Build history of the part. All positions in model axes, mm. Face numbers are marked on the shaded views. A direction names the side the tool comes from. Round coordinates to 2 decimals unless told otherwise and drop trailing zeros. Write each loop counter-clockwise with the first axis right and the second up, starting at its lowest first coordinate (ties: lowest second). Pieces come first, ordered by that corner, then holes. Notation, with made-up numbers: (86.5, 2.25) -> (138.5, 2.25) arc R24 ccw to (138.5, 15.25) -> close; hole circle Ø11 at (40.25, -15.75). An arc over 180 degrees is marked (long way). Return JSON: item names as keys, results as strings.
from build123d import *

# Parameters (mm, degrees)
BOSS_EXTRUDE1_DEPTH = 2.9591
SWEEP1_PROFILE_R    = 2.9591
SWEEP2_PROFILE_R    = 2.9591


with BuildPart() as part:
    # Sketch1 → Boss-Extrude1 (new, symmetric)
    with BuildSketch(Plane(origin=(0, 0, 0), x_dir=(1, 0, 0), z_dir=(0, 1, 0))):
        Polygon((7.97759508, 13.8176), (-7.97759508, 13.8176), (-15.955190159, 0), (-7.97759508, -13.8176), (7.97759508, -13.8176), (15.955190159, 0), align=None)
        Polygon((8.62284174, 0), (4.31142087, 7.4676), (-4.31142087, 7.4676), (-8.62284174, 0), (-4.31142087, -7.4676), (4.31142087, -7.4676), align=None, mode=Mode.SUBTRACT)
    extrude(amount=BOSS_EXTRUDE1_DEPTH, both=True)

    # Sweep1: sweep along a path in Sketch6
    with BuildLine(Plane(origin=(0, 0, 0), x_dir=(1, 0, 0), z_dir=(0, 1, 0))) as sweep1_path:
        Line((0, -13.8176), (0, -49.8856))
    # Sweep1 profile (on start of the path) → Sweep1 (sweep)
    with BuildSketch(Plane.XY.offset(13.8176)):
        Circle(SWEEP1_PROFILE_R)
    sweep(path=sweep1_path.line)

    # Sweep2: sweep along a path in Sketch6<4>
    with BuildLine(Plane(origin=(0, 0, 0), x_dir=(1, 0, 0), z_dir=(0, 1, 0))) as sweep2_path:
        Line((25.4, -49.8856), (-25.4, -49.8856))
    # Sweep2 profile (on start of the path) → Sweep2 (sweep)
    with BuildSketch(Plane(origin=(25.4, 0, 49.8856), x_dir=(0, 0, -1), z_dir=(-1, 0, 0))):
        Circle(SWEEP2_PROFILE_R)
    sweep(path=sweep2_path.line)


solid = part.part
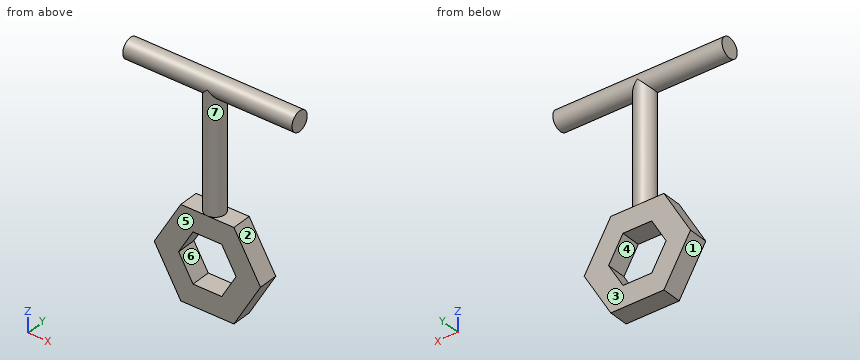
Q1. Saw through at B-B on y = 0. List the corners of the cut face in (x, z).
Verdict:
{"outline": "(-25.4, 46.93) -> (-2.96, 46.93) -> (-2.96, 13.82) -> (-7.98, 13.82) -> (-15.96, 0) -> (-7.98, -13.82) -> (7.98, -13.82) -> (15.96, 0) -> (7.98, 13.82) -> (2.96, 13.82) -> (2.96, 46.93) -> (25.4, 46.93) -> (25.4, 52.84) -> (-25.4, 52.84) -> close; hole (-8.62, 0) -> (-4.31, -7.47) -> (4.31, -7.47) -> (8.62, 0) -> (4.31, 7.47) -> (-4.31, 7.47) -> close"}
Q2. 3-axis set-ups, long thin cutter, end or side, ignore diameter. For the marked faces 5, 6 and 7: which of +Z, -Z, +X, -X, +Y, -Y reach the whole face in a straight line?
Verdict:
{"face 5": "+Z, -Z, +X, -X, -Y", "face 6": "+Y, -Y", "face 7": "none"}
Q3. Pin check, flat tips, straight feed: pin 1 Ø2 at (y, z) = (-0.5, 42) entering from -X; pin 2 Ø4 at (x, z) = (-1, 17.5) entering from -Y; pin 3 Ø2 at (y, z) = (0, -3.5) entering from +X. Stop position of each tip, or through.
Verdict:
{"pin 1": "stops at x = -2.96", "pin 2": "stops at y = -2.96", "pin 3": "stops at x = 14.51"}
Q4. Saw through at C-C on x = -1. List the corners of the cut face in (y, z) (3 decimals).
Verdict:
{"outline": "(-2.959, -13.818) -> (2.959, -13.818) -> (2.959, -7.468) -> (-2.959, -7.468) -> close; (-2.959, 7.468) -> (2.959, 7.468) -> (2.959, 13.818) -> (2.785, 13.818) -> (2.785, 48.886) arc R2.959 ccw (long way) to (-2.785, 48.886) -> (-2.785, 13.818) -> (-2.959, 13.818) -> close"}
Q5. Saw through at A-A on z = -2. List the corners of the cut face in (x, y), then the cut area to 3 significant figures.
Verdict:
{"outline": "(-14.8, -2.96) -> (-7.47, -2.96) -> (-7.47, 2.96) -> (-14.8, 2.96) -> close; (7.47, -2.96) -> (14.8, -2.96) -> (14.8, 2.96) -> (7.47, 2.96) -> close", "area": "86.8 mm²"}
Q6. Saw through at D-D on z = 38.5. List the corners of the cut face in (x, y), then the cut area to 3 significant figures.
Verdict:
{"outline": "circle Ø5.92 at (0, 0)", "area": "27.5 mm²"}
Q7. Two-plate mould, pull along X, no slides. Class the marked faces 1, 2, 3 and 4: +X half, -X half, draft (parallel to the pull), parting line (faces both ways), or undercut.
Verdict:
{"face 1": "-X half", "face 2": "+X half", "face 3": "draft", "face 4": "undercut"}
Q8. Wall check: L1, parallel to Z at x = -4, y = 1; L2, parallel to Z at x = -9.5, y = 1.55; L3, parallel to X at y = -0.15, z = 30.5. Give the ranges that are in metal, low to high.
Verdict:
{"L1": "z = -13.82 to -7.47, 7.47 to 13.82, 47.1 to 52.67", "L2": "z = -11.18 to 11.18, 47.36 to 52.41", "L3": "x = -2.96 to 2.96"}
